from build123d import *

# Parameters (mm, degrees)
BOSS_EXTRUDE1_DEPTH         = 12.7
TAP_DRILL_FOR_M6X1_0_TAP1_D = 5
FILLET1_R                   = 3


with BuildPart() as part:
    # Sketch1 → Boss-Extrude1 (new body)
    with BuildSketch(Plane(origin=(0, 0, 0), x_dir=(1, 0, 0), z_dir=(0, 1, 0))):
        with BuildLine():
            Line((-25, -15), (-25, -25))
            Line((-25, -25), (-9, -25))
            Line((-9, -25), (-9, -10.723805295))
            ThreePointArc((-9, -10.723805295), (0, 14), (9, -10.723805295))
            Line((9, -10.723805295), (9, -25))
            Line((9, -25), (25, -25))
            Line((25, -25), (25, -15))
            ThreePointArc((25, -15), (40, 0), (25, 15))
            Line((25, 15), (25, 25))
            Line((25, 25), (15, 25))
            ThreePointArc((15, 25), (0, 40), (-15, 25))
            Line((-15, 25), (-25, 25))
            Line((-25, 25), (-25, 15))
            ThreePointArc((-25, 15), (-40, 0), (-25, -15))
        make_face()
    extrude(amount=-BOSS_EXTRUDE1_DEPTH)

    # Tap Drill for M6x1.0 Tap1 (through all)
    with Locations(Plane(origin=(-15.5, 0, 15.5), x_dir=(0, 0, 1), z_dir=(0, 1, 0))):
        with Locations((0, 0), (-31, 0), (-31, 31), (0, 31), (-15.5, -14.5), (-45.5, 15.5), (-15.5, 45.5)):
            Hole(TAP_DRILL_FOR_M6X1_0_TAP1_D / 2)

    # Fillet1
    fillet1_edges = [part.edges().sort_by_distance(p)[0] for p in [
        (-25, -6.35, -15),
        (-25, -6.35, -25),
        (-15, -6.35, -25),
        (15, -6.35, -25),
        (25, -6.35, -25),
        (25, -6.35, -15),
        (25, -6.35, 15),
        (25, -6.35, 25),
        (9, -6.35, 25),
        (9, -6.35, 10.723805295),
        (-9, -6.35, 10.723805295),
        (-9, -6.35, 25),
        (-25, -6.35, 25),
        (-25, -6.35, 15),
    ]]
    fillet(fillet1_edges, radius=FILLET1_R)


solid = part.part
Model file for the job. Use its own axes, mm. A direction names the side the tool comes from. Round coordinates to 2 decimals unless told otherwise and drop trailing zeros. Order: outer loops, then holes, each group sorted by start corner. A loop starts at its lowest first (then second) coordinate and runs counter-clockwise, first axis right, second up.
(1) Band-saw the part on C-C (z = -31). List the corners of the cut face in (x, y).
(2) Pin check, flat tips, straight feed: pin 1 (4.5 mm diameter, centred on x = -30, z = 0, fed in from +Y); pin 2 (4.5 mm diameter, centred on y = -8.5, z = 20.5, fed in from -X); pin 3 (5 mm diameter, centred on y = -9.5, z = 17.5, fed in from +X); pin 4 (5 mm diameter, centred on y = -3.5, z = -5.5, fed in from +X). Stop position of each tip, or through.
(3) Band-saw the part on B-B (x = -30). List the corners of the cut face in (y, z).
(4) Drill centre lines: line 1 (X direction, y = -1.5, z = -0.5); line 2 (Z direction, x = 17, y = -2.75); line 3 (X direction, y = -0.25, z = 7.5). Where is each one in solid material? Low to high.
(5) 3-axis set-ups, long thin cutter, end or side, ignore diameter. For faces 1 (the face through (-9.22, -6.44, 10.91)), 2 (the face through (-9.9, -6.44, 24.14)), 3 (the face through (20, -6, -25)), 4 (the face through (-40, -6, 0)): which of +Z, -Z, +X, -X, +Y, -Y reach the whole face in a straight line?
(6) Pull direction X, two halves, no side cores. Call faces 5 (the face through (-1, -12.7, -15)), 6 (the face through (25.69, -6.439, 15.834)), 7 (the face through (9, -6, 17)): released by +X, released by -X, zero draft, split by the parting line, or undercut.
(7) Band-saw the part on D-D (y = -2.75). Give the number of separate pieces and of enclosed holes in the cut face, then the cut area to 3 significant figures.
(8) Band-saw the part on A-A (z = 0). List the corners of the cut face in (x, y).
Verdict:
1. outline: (-13.75, -12.7) - (-2.29, -12.7) - (-2.29, 0) - (-13.75, 0) - close; (2.29, -12.7) - (13.75, -12.7) - (13.75, 0) - (2.29, 0) - close
2. pin 1: passes through
2. pin 2: stops at x = -25
2. pin 3: stops at x = 26.8
2. pin 4: stops at x = 39.7
3. outline: (-12.7, -14.14) - (0, -14.14) - (0, -2.5) - (-12.7, -2.5) - close; (-12.7, 2.5) - (0, 2.5) - (0, 14.14) - (-12.7, 14.14) - close
4. line 1: x = -39.99 to -32.45, -27.55 to -13.99, 13.99 to 27.55, 32.45 to 39.99
4. line 2: z = -25.09 to -17.5, -13.5 to 13.5, 17.5 to 25
4. line 3: x = -37.99 to -11.82, 11.82 to 37.99
5. face 1: +Y, -Y
5. face 2: +Z, +Y, -Y
5. face 3: -Z, +X, +Y, -Y
5. face 4: -X, +Y, -Y
6. face 5: zero draft
6. face 6: released by +X
6. face 7: undercut
7. separate pieces: 1
7. enclosed holes: 7
7. area: 2,590 mm2
8. outline: (-40, -12.7) - (-32.5, -12.7) - (-32.5, 0) - (-40, 0) - close; (-27.5, -12.7) - (-14, -12.7) - (-14, 0) - (-27.5, 0) - close; (14, -12.7) - (27.5, -12.7) - (27.5, 0) - (14, 0) - close; (32.5, -12.7) - (40, -12.7) - (40, 0) - (32.5, 0) - close
